from build123d import *

# Parameters (mm, degrees)
SKETCH1_R           = 15
BOSS_EXTRUDE1_DEPTH = 200
SKETCH2_R           = 30
SKETCH2_R_2         = 15
BOSS_EXTRUDE2_DEPTH = 70
CUT_EXTRUDE1_DEPTH  = 84
CIRPATTERN2_COUNT   = 3


with BuildPart() as part:
    # Sketch1 → Boss-Extrude1 (new body)
    with BuildSketch(Plane(origin=(0, 0, 0), x_dir=(1, 0, 0), z_dir=(0, 1, 0))):
        Circle(SKETCH1_R)
    extrude(amount=BOSS_EXTRUDE1_DEPTH)

    # Sketch2 → Boss-Extrude2 (add)
    with BuildSketch(Plane.XZ):
        Circle(SKETCH2_R)
        Circle(SKETCH2_R_2, mode=Mode.SUBTRACT)
    extrude(amount=-BOSS_EXTRUDE2_DEPTH)

    # Sketch3 → Cut-Extrude1 (cut)
    with BuildSketch(Plane(origin=(0, 70, 0), x_dir=(1, 0, 0), z_dir=(0, 1, 0))):
        Polygon((-3.333611713, -14.624877194), (-7.415359219, -32.531898508), (7.415359219, -32.531898508), (3.333611713, -14.624877194), (0, -15), align=None)
    cut_extrude1 = extrude(amount=-CUT_EXTRUDE1_DEPTH, mode=Mode.SUBTRACT)

    # CirPattern2: Cut-Extrude1 ×3 about axis
    cirpattern2_axis = Axis((0, 0, 0), (0, 1, 0))
    for i in range(1, CIRPATTERN2_COUNT):
        add(cut_extrude1.rotate(cirpattern2_axis, i * 360 / CIRPATTERN2_COUNT), mode=Mode.SUBTRACT)


solid = part.part
Source: CAD feature listing. Evaluate the final solid. Frame: model axes, mm. A direction names the side the tool comes from. Round coordinates to 2 decimals unless told otherwise and drop trailing zeros. Write each loop counter-clockwise with the first axis right and the second up, starting at its lowest first coordinate (ties: lowest second). Pieces come first, ordered by that corner, then holes. Notation, with made-up numbers: M 70.5,-3 L 98.5,-3 A27 cw 98.5,15 Z; hole C -12.5,58.5 d7. An arc over 180 degrees is marked long. One line per item, written item: value. Start each with the question number.
Item 1: Pin query (flat end, axial travel): pin 1 (6 mm diameter, centred on y = 83, z = -4.5, fed in from -X); pin 2 (12 mm diameter, centred on y = 174.5, z = 1, fed in from -X); pin 3 (5 mm diameter, centred on x = 13, z = 23, fed in from +Y). Return the tip coordinate at first contact, or that it passes through.
Item 2: Set-up query: faces 1 (the cylindrical face through (-14.985, 134.09, -0.66)), 2 (the flat face through (-4.977, 35.49, 21.835)), 3 (the flat face through (21.398, 35.49, -6.607)), 4 (the flat face through (-16.421, 35.49, -15.228)). Return all of +Z, -Z, +X, -X, +Y, -Y with unobstructed straight access to the full face (end or side cutting, diameter ignored); none if empty.
Item 3: Section query A-A (y = 21). Return the cut outline in (x, z), plus the area to 3 significant figures.
Item 4: Section query B-B (z = 23.5). Return the cut outline in (x, y), plus the area to 3 significant figures.
Item 5: Section query C-C (z = 0). Return the cut outline in (x, y).
Item 6: Section query D-D (y = 136). Return the cut outline in (x, z).
Item 7: Mould query, pull axis Z, two halves, no side actions, for faces 5 (the flat face through (-21.6, 35.49, -6.67)), 6 (the flat face through (0, 200, 0)), 7 (the cylindrical face through (0, 35, -30)). Classes: pulls with the +Z half, pulls with the -Z half, needs draft (parallel to the pull), parting line crosses it, or undercut.
Item 8: Ray query, L1, parallel to Y at x = 15, z = 8.5; L2, parallel to Z at x = 14, y = 18.5; L3, parallel to X at y = 23, z = 22. Return the intervals inside material, ascending. Write a range as from..to.
Result set:
1. pin 1: stops at x = -14.92
1. pin 2: stops at x = -15
1. pin 3: stops at y = 70
2. face 1: +Y
2. face 2: +Z, +Y, -Y
2. face 3: +Y, -Y
2. face 4: -X, +Y, -Y
3. outline: M -28.66,-8.85 L -14.33,-4.43 L -12.99,-7.5 L -11,-10.2 L -22,-20.4 A30 ccw 22,-20.4 L 11,-10.2 L 12.99,-7.5 L 14.33,-4.43 L 28.66,-8.85 A30 ccw 6.67,29.25 L 3.33,14.62 L 0,15 L -3.33,14.62 L -6.67,29.25 A30 ccw Z
3. area: 2,370 mm²
4. outline: M -18.65,0 L -5.36,0 L -5.36,70 L -18.65,70 Z; M 5.36,0 L 18.65,0 L 18.65,70 L 5.36,70 Z
4. area: 1,860 mm²
5. outline: M -30,0 L 30,0 L 30,70 L 15,70 L 15,200 L -15,200 L -15,70 L -30,70 Z
6. outline: C 0,0 d30
7. face 5: undercut
7. face 6: needs draft
7. face 7: pulls with the -Z half
8. L1: y = 0..70
8. L2: z = -26.53..-12.98, -5.19..26.53
8. L3: x = -20.4..-5.01, 5.01..20.4
